```python
from build123d import *
from build123d import SkipClean  # not in build123d's __all__

# Parameters (mm, degrees)
F0_R     = 3.175
F0_R_2   = 9.525
F1_DEPTH = 25.4


# Not quite as in the source:
# - a pattern or mirror of a feature is missing from the dataset's text; its kind, count and spacing are read off the source's solid


with BuildPart() as f1:
    # F0 (on Top) → F1 (new body)
    with BuildSketch(Plane.XY):
        with BuildLine():
            Line((0, 38.1), (-114.3, 38.1))
            Line((-114.3, 38.1), (-114.3, -38.1))
            Line((-114.3, -38.1), (0, -38.1))
            Line((0, -38.1), (0, -6.35))
            ThreePointArc((0, -6.35), (-6.35, 0), (0, 6.35))
            Line((0, 6.35), (0, 38.1))
        make_face()
        with Locations((-76.2, -26.543)):
            Circle(F0_R, mode=Mode.SUBTRACT)
        with Locations((-102.743, 0)):
            Circle(F0_R, mode=Mode.SUBTRACT)
        with Locations((-76.2, 0)):
            Circle(F0_R_2, mode=Mode.SUBTRACT)
        with Locations((-76.2, 26.543)):
            Circle(F0_R, mode=Mode.SUBTRACT)
        with Locations((-49.657, 0)):
            Circle(F0_R, mode=Mode.SUBTRACT)
    extrude(amount=F1_DEPTH)

    # F1_copies: F1 across plane


with BuildPart() as f1_1:
    add(f1.part, clean=False)
    with SkipClean():  # cleaning this boolean's faces spoils the solid; the shape is the same uncleaned
        add(f1.part.mirror(Plane(origin=(0, 0, 0), x_dir=(0, 0, 1), z_dir=(1, 0, 0))), clean=False)


solid = f1_1.part
```
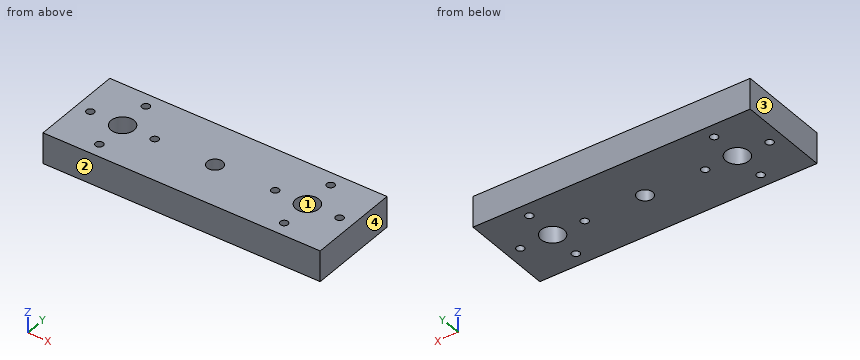
Can you work these out from the model? Positions are in its coordinate system, mm. Face numbers are marked on the shaded views. Round coordinates to 2 decimals unless told otherwise and drop trailing zeros. Loops run counter-clockwise (first coordinate to the right, second up) from the corner with the lowest first, then second, coordinate; pieces in that order, holes last. Notation, with made-up numbers: M -32,-26.5 L 1,-26.5 A19 cw 1,-6.5 Z; hole C 86,16.25 d10. An arc over 180 degrees is marked long. Answer as a JSON object with one key per item and string values. Group by question number.
Q1. We'd pull the mould along X, two halves only. Please class the marked faces 1, 2, 3 and 4: +X half, -X half, draft (parallel to the pull), parting line (faces both ways), or undercut.
Q2. Please list where these lines run through material, in increasing order: L1, parallel to X at y = 27, z = 12.25; L2, parallel to X at y = 26.5, z = 5.25; L3, parallel to Y at x = 76.2, z = 11.5 (3 decimals).
Q3. Imagine slicing it at B-B, the plane x = 76.2. Please give me the cut outline in (y, z) (3 decimals).
Q4. Will this pin go through, and if not, where does the flat tip stop? pin 1 (4 mm diameter, centred on x = 49.657, y = 0, fed in from -Z).
Q5. Imagine slicing it at A-A, the plane x = 0. Please give me the cut outline in (y, z), then the cut area to 3 significant figures.
Q6. Imagine slicing it at C-C, the plane y = 0. Count the separate pieces of the cut face and the enclosed holes in it, then the cut area to 3 significant figures.
Findings:
{
 "1": {"face 1": "undercut", "face 2": "draft", "face 3": "-X half", "face 4": "+X half"},
 "2": {"L1": "x = -114.3 to -79.34, -73.06 to 73.06, 79.34 to 114.3", "L2": "x = -114.3 to -79.37, -73.03 to 73.03, 79.37 to 114.3", "L3": "y = -38.1 to -29.718, -23.368 to -9.525, 9.525 to 23.368, 29.718 to 38.1"},
 "3": {"outline": "M -38.1,0 L -29.718,0 L -29.718,25.4 L -38.1,25.4 Z; M -23.368,0 L -9.525,0 L -9.525,25.4 L -23.368,25.4 Z; M 9.525,0 L 23.368,0 L 23.368,25.4 L 9.525,25.4 Z; M 29.718,0 L 38.1,0 L 38.1,25.4 L 29.718,25.4 Z"},
 "4": {"pin 1": "passes through"},
 "5": {"outline": "M -38.1,0 L -6.35,0 L -6.35,25.4 L -38.1,25.4 Z; M 6.35,0 L 38.1,0 L 38.1,25.4 L 6.35,25.4 Z", "area": "1,610 mm2"},
 "6": {"separate pieces": "8", "enclosed holes": "0", "area": "3,870 mm2"}
}
